```python
from build123d import *

# Parameters (mm, degrees)
SKETCH1_W                                        = 1174.75
SKETCH1_H                                        = 749.3
SKETCH1_W_2                                      = 711.2
SKETCH1_H_2                                      = 508
BOSS_EXTRUDE1_DEPTH                              = 12.7
FILLET1_R                                        = 101.6
CSK_FOR_1_4_FLAT_HEAD_MACHINE_SCREW1_D           = 6.7564
CSK_FOR_1_4_FLAT_HEAD_MACHINE_SCREW1_CSINK_D     = 12.8778
CSK_FOR_1_4_FLAT_HEAD_MACHINE_SCREW1_CSINK_ANGLE = 82
FILLET2_R                                        = 25.4


with BuildPart() as part:
    # Sketch1 → Boss-Extrude1 (new body)
    with BuildSketch(Plane.XY):
        Rectangle(SKETCH1_W, SKETCH1_H)
        Rectangle(SKETCH1_W_2, SKETCH1_H_2, mode=Mode.SUBTRACT)
    extrude(amount=BOSS_EXTRUDE1_DEPTH)

    # Fillet1
    fillet1_edges = [part.edges().sort_by_distance(p)[0] for p in [
        (355.6, -254, 6.35),
        (355.6, 254, 6.35),
        (-355.6, 254, 6.35),
        (-355.6, -254, 6.35),
    ]]
    fillet(fillet1_edges, radius=FILLET1_R)

    # CSK for 1/4 Flat Head Machine Screw1 (through all)
    with Locations(Plane.XY.offset(12.7)):
        with Locations((-568.325, -347.218), (-568.325, 0), (-377.825, 355.6), (-377.825, -355.6), (-568.325, 347.218), (377.825, -355.6), (568.325, -347.218), (568.325, 0), (568.325, 347.218), (377.825, 355.6), (-117.475, -276.225), (-117.475, 276.225), (117.475, 276.225), (117.475, -276.225)):
            CounterSinkHole(CSK_FOR_1_4_FLAT_HEAD_MACHINE_SCREW1_D / 2, CSK_FOR_1_4_FLAT_HEAD_MACHINE_SCREW1_CSINK_D / 2, counter_sink_angle=CSK_FOR_1_4_FLAT_HEAD_MACHINE_SCREW1_CSINK_ANGLE)

    # Fillet2
    fillet2_edges = [part.edges().sort_by_distance(p)[0] for p in [
        (587.375, -374.65, 6.35),
        (-587.375, -374.65, 6.35),
        (-587.375, 374.65, 6.35),
        (587.375, 374.65, 6.35),
    ]]
    fillet(fillet2_edges, radius=FILLET2_R)


solid = part.part
```
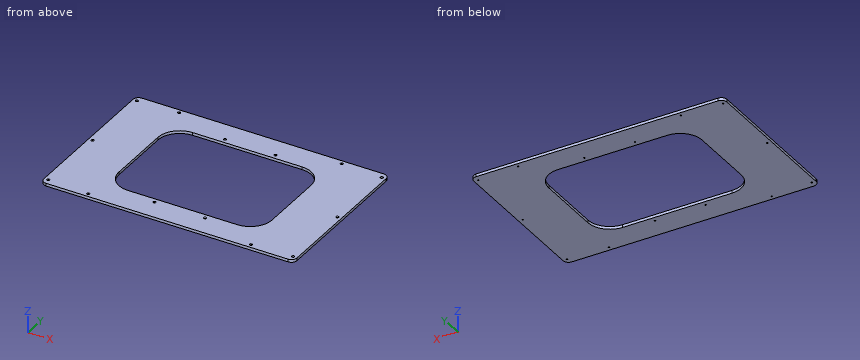
Can you work these out from the model? Positions are in its coordinate system, mm. Give positions to 0.01 mm unless a question says otherwise; leave off trailing zeros. Loops run counter-clockwise (first coordinate to the right, second up) from the corner with the lowest first, then second, coordinate; pieces in that order, holes last. Notation, with made-up numbers: M 30.5,52 L 60.5,52 A15 ccw 60.5,59 Z; hole C 12,-10.75 d4. An arc over 180 degrees is marked long. One line per item, written item: value.
(1) Suppose I cut it at B-B on x = 338. List the corners of the cut face in (y, z) for me, plus the area to 3 significant figures.
Returned:
outline: M -374.65,0 L -209.55,0 L -209.55,12.7 L -374.65,12.7 Z; M 209.55,0 L 374.65,0 L 374.65,12.7 L 209.55,12.7 Z
area: 4,190 mm^2
(2) Will these pins go through, and if not, where does the flat tip stop? pin 1 (5.5 mm diameter, centred on x = 377.825, y = -355.6, fed in from -Z); pin 2 (8 mm diameter, centred on x = -117.475, y = 276.225, fed in from +Z); pin 3 (9 mm diameter, centred on x = -377.825, y = -355.6, fed in from +Z).
Returned:
pin 1: through
pin 2: z = 9.89
pin 3: z = 10.47
(3) Suppose I cut it at C-C on z = 5.25. Count the separate pieces of the cut face and the enclosed holes in it, plus the area to 3 significant figures.
Returned:
separate pieces: 1
enclosed holes: 15
area: 527,000 mm^2
(4) Suppose I cut it at A-A on y = 82. List the corners of the cut face in (x, z) for me (3 decimals), plus the area to 3 significant figures.
Returned:
outline: M -587.375,0 L -355.6,0 L -355.6,12.7 L -587.375,12.7 Z; M 355.6,0 L 587.375,0 L 587.375,12.7 L 355.6,12.7 Z
area: 5,890 mm^2
(5) I need wall thicknesses on line 1 (X direction, y = 34.5, z = 7.5) (3 decimals); line 2 (X direction, y = 0, z = 6) (3 decimals); line 3 (X direction, y = 171.5, z = 6.5) (3 decimals). Which ranges of each line are inside material? Lowest first, please.
Returned:
line 1: -587.375 to -355.6, 355.6 to 587.375
line 2: -587.375 to -571.703, -564.947 to -355.6, 355.6 to 564.947, 571.703 to 587.375
line 3: -587.375 to -353.789, 353.789 to 587.375
